from build123d import *

# Parameters (mm, degrees)
EXTRUDE_1_DEPTH     = 5.2
EXTRUDE_2_DEPTH     = 6
EXTRUDE_START       = -11.2
EXTRUDE_3_DEPTH     = 11.2
FILLET_1_R          = 5
SKETCH_4_R          = 1.6
CUT_EXTRUDE_1_DEPTH = 22.789045413
SKETCH_7_W          = 7
SKETCH_7_H          = 3
EXTRUDE_5_DEPTH     = 8
SKETCH_8_R          = 1.45
CUT_EXTRUDE_3_DEPTH = 8
EXTRUDE_START_2     = 1
SKETCH_9_R          = 1.45
SKETCH_9_R_2        = 1.6
EXTRUDE_6_DEPTH     = 1
FILLET_2_R          = 3
FILLET_3_R          = 1
SKETCH_10_R         = 2.9
CUT_EXTRUDE_4_DEPTH = 2.7
CHAMFER_2_SIZE      = 1.3
CHAMFER_1_SIZE      = 0.4
CUT_EXTRUDE_5_DEPTH = 0.4


# Some blends are built 0.0001 mm under size
with BuildPart() as part:
    # 草图1 → 凸台-拉伸1 (new body)
    with BuildSketch(Plane(origin=(0, 0, 0), x_dir=(1, 0, 0), z_dir=(0, 1, 0))):
        with BuildLine():
            Line((-11.15, 0), (-8.15, 0))
            ThreePointArc((-8.15, 0), (0, -8.15), (8.15, 0))
            Line((8.15, 0), (11.15, 0))
            ThreePointArc((11.15, 0), (0, -11.15), (-11.15, 0))
        make_face()
    extrude(amount=EXTRUDE_1_DEPTH)

    # 草图2 → 凸台-拉伸2 (add)
    with BuildSketch(Plane(origin=(0, 5.2, 0), x_dir=(1, 0, 0), z_dir=(0, 1, 0))):
        with BuildLine():
            Line((-11.15, 0), (-6.15, 0))
            ThreePointArc((-6.15, 0), (0, -6.15), (6.15, 0))
            Line((6.15, 0), (11.15, 0))
            ThreePointArc((11.15, 0), (0, -11.15), (-11.15, 0))
        make_face()
    extrude(amount=EXTRUDE_2_DEPTH)

    # 草图3 → 凸台-拉伸3 (add)
    with BuildSketch(Plane(origin=(0, 11.2, 0), x_dir=(1, 0, 0), z_dir=(0, 1, 0)).offset(EXTRUDE_START)):
        with BuildLine():
            Line((3.911521443, -7.15), (15, -7.15))
            Line((15, -7.15), (15, -11.15))
            Line((15, -11.15), (-15, -11.15))
            Line((-15, -11.15), (-15, -7.15))
            Line((-15, -7.15), (-3.911521443, -7.15))
            ThreePointArc((-3.911521443, -7.15), (0, -8.15), (3.911521443, -7.15))
        make_face()
    extrude(amount=EXTRUDE_3_DEPTH)

    # 圆角1
    # the kernel refuses this fillet: 5 mm, written as the material it adds along each edge
    with BuildSketch(Plane(origin=(-8.555699854, 11.2, 7.15), x_dir=(-0.4058769598957605, 0, -0.9139277287760642), z_dir=(0, -1, 0))) as fillet_1_piece_1:
        with BuildLine():
            CenterArc((7.497147581, -4.807763049), FILLET_1_R, 105.939417034, 86.556633096)
            Line((2.615592952, -5.889624596), (2.517961859, -5.911261826))
            ThreePointArc((2.517961859, -5.911261826), (1.216403703, -2.985399994), (-0.091392773, -0.040587696))
            Line((-0.091392773, -0.040587696), (0.027462079, 0.096155261))
            ThreePointArc((0.027462079, 0.096155261), (3.062021814, -0.328688401), (6.096581549, 0.096155261))
            Line((6.096581549, 0.096155261), (6.124043628, 0))
        make_face()
    extrude(amount=11.2)
    with BuildSketch(Plane(origin=(8.555699854, 11.2, 7.15), x_dir=(1, 0, 0), z_dir=(0, -1, 0))) as fillet_1_piece_2:
        with BuildLine():
            CenterArc((7.436867432, -4.90049081), FILLET_1_R, 101.450043509, 86.556633096)
            Line((2.48560821, -5.596933284), (2.386583026, -5.610862133))
            ThreePointArc((2.386583026, -5.610862133), (1.543201548, -2.665059593), (-0.076732734, -0.064125561))
            Line((-0.076732734, -0.064125561), (0, 0.1))
            ThreePointArc((0, 0.1), (3.222150073, 0.1), (6.4244488, 0.098009816))
            Line((6.4244488, 0.098009816), (6.444300146, 0))
        make_face()
    extrude(amount=11.2)

    # 草图4 → 切除-拉伸1 (cut, through all)
    with BuildSketch(Plane.XY.offset(11.15)):
        with Locations((-11, 5.6)):
            Circle(SKETCH_4_R)
        with Locations((11, 5.6)):
            Circle(SKETCH_4_R)
    extrude(amount=-CUT_EXTRUDE_1_DEPTH, mode=Mode.SUBTRACT)

    # 草图7 → 凸台-拉伸5 (add)
    with BuildSketch(Plane(origin=(0, 11.2, 0), x_dir=(1, 0, 0), z_dir=(0, 1, 0))):
        with Locations((-11.5, -9.65)):
            Rectangle(SKETCH_7_W, SKETCH_7_H)
        with Locations((11.5, -9.65)):
            Rectangle(SKETCH_7_W, SKETCH_7_H)
    extrude(amount=EXTRUDE_5_DEPTH)

    # 草图8 → 切除-拉伸3 (cut)
    with BuildSketch(Plane.XY.offset(11.15)):
        with Locations((-12, 16.6)):
            Circle(SKETCH_8_R)
        with Locations((12, 16.6)):
            Circle(SKETCH_8_R)
    extrude(amount=-CUT_EXTRUDE_3_DEPTH, mode=Mode.SUBTRACT)

    # 草图9 → 凸台-拉伸6 (add)
    with BuildSketch(Plane.XY.offset(11.15).offset(EXTRUDE_START_2)):
        Polygon((-15, 19.2), (-15, 0), (15, 0), (15, 19.2), (8, 19.2), (8, 11.2), (-8, 11.2), (-8, 19.2), align=None)
        with Locations((-12, 16.6)):
            Circle(SKETCH_9_R, mode=Mode.SUBTRACT)
        with Locations((-11, 5.6)):
            Circle(SKETCH_9_R_2, mode=Mode.SUBTRACT)
        with Locations((11, 5.6)):
            Circle(SKETCH_9_R_2, mode=Mode.SUBTRACT)
        with Locations((12, 16.6)):
            Circle(SKETCH_9_R, mode=Mode.SUBTRACT)
    extrude(amount=-EXTRUDE_6_DEPTH)

    # 圆角2
    fillet_2_edges = [part.edges().sort_by_distance(p)[0] for p in [
        (8, 11.2, 10.15),
        (-8, 11.2, 10.15),
    ]]
    fillet(fillet_2_edges, radius=FILLET_2_R)

    # 圆角3
    fillet_3_edges = [part.edges().sort_by_distance(p)[0] for p in [
        (15, 19.2, 10.15),
        (8, 19.2, 10.15),
        (-15, 19.2, 10.15),
        (-8, 19.2, 10.15),
    ]]
    fillet(fillet_3_edges, radius=FILLET_3_R)

    # 草图10 → 切除-拉伸4 (cut)
    with BuildSketch(Plane.XY.offset(12.15)):
        with Locations((-11, 5.6)):
            Circle(SKETCH_10_R)
        with Locations((11, 5.6)):
            Circle(SKETCH_10_R)
    extrude(amount=-CUT_EXTRUDE_4_DEPTH, mode=Mode.SUBTRACT)

    # 倒角2
    chamfer_2_edges = [part.edges().sort_by_distance(p)[0] for p in [
        (-13.9, 5.6, 9.45),
        (8.1, 5.6, 9.45),
    ]]
    chamfer(chamfer_2_edges, length=CHAMFER_2_SIZE - 0.0001)  # a hair under: the kernel refuses the full size

    # 倒角1
    chamfer_1_edges = [part.edges().sort_by_distance(p)[0] for p in [
        (0, 0, 12.15),
        (15, 9.1, 12.15),
        (-13.45, 16.6, 12.15),
        (10.55, 16.6, 12.15),
        (0, 11.2, 12.15),
        (-8, 16.2, 12.15),
        (7.121320344, 12.078679656, 12.15),
        (-7.121320344, 12.078679656, 12.15),
        (11.5, 19.2, 12.15),
        (-11.5, 19.2, 12.15),
        (-15, 9.1, 12.15),
        (8, 16.2, 12.15),
        (-14.707106781, 18.907106781, 12.15),
        (-8.292893219, 18.907106781, 12.15),
        (8.292893219, 18.907106781, 12.15),
        (14.707106781, 18.907106781, 12.15),
        (-13.9, 5.6, 12.15),
        (8.1, 5.6, 12.15),
    ]]
    chamfer(chamfer_1_edges, length=CHAMFER_1_SIZE)

    # 草图11 → 切除-拉伸5 (cut)
    with BuildSketch(Plane(origin=(0, 0, 8.15), x_dir=(-1, 0, 0), z_dir=(0, 0, -1))):
        Polygon((-8.709103466, 16.6), (-10.354551733, 19.45), (-13.645448267, 19.45), (-15.290896534, 16.6), (-13.645448267, 13.75), (-10.354551733, 13.75), align=None)
        Polygon((15.290896534, 16.6), (13.645448267, 19.45), (10.354551733, 19.45), (8.709103466, 16.6), (10.354551733, 13.75), (13.645448267, 13.75), align=None)
    extrude(amount=-CUT_EXTRUDE_5_DEPTH, mode=Mode.SUBTRACT)


solid = part.part
Geometry check sheet. Reference: the model listing, model coordinates, mm. A direction names the side the tool comes from. Give positions to 0.01 mm unless a question says otherwise; leave off trailing zeros. Order: outer loops, then holes, each group sorted by start corner. A loop starts at its lowest first (then second) coordinate and runs counter-clockwise, first axis right, second up.
1) Draft check along Y on faces 1 (the cylindrical face through (-13.301, 3.835, 11.257)), 2 (the cylindrical face through (-0.14, 8.16, 6.15)), 3 (the cylindrical face through (-7.14, 12.1, 9.92)). Enter one of: released by +Y, released by -Y, zero draft, split by the parting line, or undercut.
Results are:
face 1: undercut
face 2: zero draft
face 3: released by +Y
2) Cross-section at D-D (y = 17.5). Give the number of separate pieces and of enclosed holes in the cut face, then the cut area to 3 significant figures.
Results are:
separate pieces: 4
enclosed holes: 0
area: 34.5 mm2
3) Tool access check on faces 4 (the flat face through (-9.52, 15.195, 8.347)), 5 (the flat face through (14.6, 18.4, 8.15)), 6 (the flat face through (0, 5.2, 6.5)), 7 (the cylindrical face through (7.14, 12.1, 9.92)). Record the directions out of +Z, -Z, +X, -X, +Y, -Y that give a thin tool (end or side, any length) a straight path to the whole face; none if there is none.
Results are:
face 4: -Z
face 5: -Z, +X, -X, +Y
face 6: -Z, -Y
face 7: +Z, -Z, +Y
4) Gauge pin test, flat ends, axial feed: pin 1 (4 mm diameter, centred on x = -11, y = 5.6, fed in from +Z); pin 2 (6 mm diameter, centred on x = -10.5, y = 15.5, fed in from -Z); pin 3 (2 mm diameter, centred on y = 10.5, z = 5.5, fed in from +X). Record the tip position at first contact, or that the pin passes through.
Results are:
pin 1: stops at z = 9.85
pin 2: stops at z = 8.15
pin 3: stops at x = 13.36
5) Material ranges on probe 1 along Y at (x, z) = (-12, 10.4); probe 2 along Y at (x, z) = (11, 11.55); probe 3 along Z at (x, y) = (-10.5, 12), recorded low to high.
Results are:
probe 1: y = 0 to 3.25, 7.95 to 15.15, 18.05 to 19.2
probe 2: y = 0 to 2.7, 8.5 to 15.55, 17.65 to 19.2
probe 3: z = 8.15 to 12.15
6) Cross-section at A-A (z = 2.75). Record the boundary of the cut face in (x, y), then the cut area to 3 significant figures.
Results are:
outline: (-11.02, 0) - (-7.67, 0) - (-7.67, 5.2) - (-5.5, 5.2) - (-5.5, 11.2) - (-11.02, 11.2) - (-11.02, 7.2) arc R1.6 cw (long way) to (-11.02, 4) - close; (5.5, 5.2) - (7.67, 5.2) - (7.67, 0) - (11.02, 0) - (11.02, 4) arc R1.6 cw (long way) to (11.02, 7.2) - (11.02, 11.2) - (5.5, 11.2) - close
area: 92.8 mm2
7) Cross-section at B-B (x = 0). Record the boundary of the cut face in (y, z), then the cut area to 3 significant figures.
Results are:
outline: (0, 8.15) - (5.2, 8.15) - (5.2, 6.15) - (11.2, 6.15) - (11.2, 11.75) - (10.8, 12.15) - (0.4, 12.15) - (0, 11.75) - close
area: 56.6 mm2
8) Cross-section at C-C (z = 6.5). Record the boundary of the cut face in (x, y), then the cut area to 3 significant figures.
Results are:
outline: (-13.36, 0) - (-4.92, 0) - (-4.92, 5.2) - (4.92, 5.2) - (4.92, 0) - (13.36, 0) - (13.36, 11.2) - (-13.36, 11.2) - close; hole circle Ø3.2 at (-11, 5.6); hole circle Ø3.2 at (11, 5.6)
area: 232 mm2
